The model under review builds one solid part; all positions refer to its coordinate system, in mm. A direction names the side the tool comes from. Give positions to 0.01 mm unless a question says otherwise; leave off trailing zeros. Order: outer loops, then holes, each group sorted by start corner. A loop starts at its lowest first (then second) coordinate and runs counter-clockwise, first axis right, second up. Notation, with made-up numbers: (6, 68) - (65, 68) arc R31 ccw to (65, 97) - close; hole circle Ø3 at (36.25, 48). An arc over 180 degrees is marked (long way). Put each result on its own line as item: value.
```python
from build123d import *

# Parameters (mm, degrees)
F1_DEPTH = 25.4
F3_DEPTH = 25.401


with BuildPart() as f1:
    # F0 (on Front) → F1 (new body)
    with BuildSketch(Plane.XZ):
        Polygon((2.206567, 32.044211), (0, 32.044211), (0, 0), (38.1, 0), (38.1, 31.75), align=None)
    extrude(amount=F1_DEPTH)

    # F2 (on Front) → F3 (cut, through all)
    with BuildSketch(Plane.XZ):
        Polygon((25.766958, 9.347903), (38.466958, 9.347903), (37.892044, 31.662248), (12.7, 31.662248), align=None)
    extrude(amount=F3_DEPTH, mode=Mode.SUBTRACT)


solid = f1.part
```
(1) The part is to be moulded in two halves that separate along Z. For faces 1 (the flat face through (15, -25.4, 13)), 2 (the flat face through (19, -13, 0)), 3 (the flat face through (32, -13, 9.348)), say which applies: pulls with the +Z half, pulls with the -Z half, needs draft (parallel to the pull), parting line crosses it, or undercut.
The answers:
face 1: needs draft
face 2: pulls with the -Z half
face 3: undercut
(2) Take a section at B-B, the plane y = -11.25. Write out the cut boundary in (x, z).
The answers:
outline: (0, 0) - (38.1, 0) - (38.1, 9.35) - (25.77, 9.35) - (12.7, 31.66) - (37.89, 31.66) - (38.1, 23.59) - (38.1, 31.75) - (2.21, 32.04) - (0, 32.04) - close
(3) Clearance check with flat-ended pins moving along their axes: pin 1 Ø10 at (x, y) = (34, -8.5) entering from +Z; pin 2 Ø8 at (x, y) = (8, -15) entering from +Z. State where each tip first meets the part, or that it passes through.
The answers:
pin 1: z = 31.82
pin 2: z = 32.03
(4) Take a section at A-A, the plane x = 35. Write out the cut boundary in (y, z), then the cut area to 3 significant figures.
The answers:
outline: (-25.4, 0) - (0, 0) - (0, 9.35) - (-25.4, 9.35) - close; (-25.4, 31.66) - (0, 31.66) - (0, 31.78) - (-25.4, 31.78) - close
area: 240 mm^2
(5) For faces 4 (the flat face through (0, -13, 16)), 5 (the flat face through (25, -13, 31.662)), list the 3-axis set-ups (+Z, -Z, +X, -X, +Y, -Y) from which the entire face can be reached by the end or side of a thin tool; tool diameter is ignored.
The answers:
face 4: +Z, -Z, -X, +Y, -Y
face 5: +Y, -Y
(6) Take a section at D-D, the plane z = 20. Write out the cut boundary in (x, y), then the cut area to 3 significant figures.
The answers:
outline: (0, -25.4) - (19.53, -25.4) - (19.53, 0) - (0, 0) - close
area: 496 mm^2
(7) Take a section at C-C, the plane z = 27.5. Write out the cut boundary in (x, y).
The answers:
outline: (0, -25.4) - (15.14, -25.4) - (15.14, 0) - (0, 0) - close; (38, -25.4) - (38.1, -25.4) - (38.1, 0) - (38, 0) - close
(8) Wall thickness on L1, parallel to X at y = -23.75, z = 30.5; L2, parallel to Z at x = 13, y = -11; L3, parallel to Z at x = 24, y = -4: over which ranges is each line inside the solid? List them lowest first.
The answers:
L1: 0 to 13.38, 37.92 to 38.1
L2: 0 to 31.15, 31.66 to 31.96
L3: 0 to 12.37, 31.66 to 31.87
